```python
from build123d import *

# Parameters (mm, degrees)
SKETCH1_W           = 90
SKETCH1_H           = 145
BOSS_EXTRUDE2_DEPTH = 10
FILLET2_R           = 20
BOSS_EXTRUDE6_DEPTH = 60
CUT_EXTRUDE1_START  = -45
CUT_EXTRUDE1_DEPTH  = 30
SKETCH13_R          = 12
CUT_EXTRUDE2_DEPTH  = 127
BOSS_EXTRUDE8_DEPTH = 10
SKETCH17_R          = 9
CUT_EXTRUDE3_DEPTH  = 20


with BuildPart() as part:
    # Sketch1 → Boss-Extrude2 (new, symmetric)
    with BuildSketch(Plane(origin=(0, 0, 0), x_dir=(1, 0, 0), z_dir=(0, 1, 0))):
        Rectangle(SKETCH1_W, SKETCH1_H)
    extrude(amount=BOSS_EXTRUDE2_DEPTH, both=True)

    # Fillet2
    fillet2_edges = [part.edges().sort_by_distance(p)[0] for p in [
        (45, 0, -72.5),
        (45, 0, 72.5),
        (-45, 0, 72.5),
        (-45, 0, -72.5),
    ]]
    fillet(fillet2_edges, radius=FILLET2_R)

    # Sketch8 → Boss-Extrude6 (add)
    with BuildSketch(Plane(origin=(0, 10, 0), x_dir=(1, 0, 0), z_dir=(0, 1, 0))):
        with BuildLine():
            Line((-34, -7.5), (-34, 42.5))
            ThreePointArc((-34, 42.5), (0, 76.5), (34, 42.5))
            Line((34, 42.5), (34, -7.5))
            Line((34, -7.5), (-34, -7.5))
        make_face()
    extrude(amount=BOSS_EXTRUDE6_DEPTH)

    # Sketch9 → Cut-Extrude1 (cut)
    with BuildSketch(Plane(origin=(0, 70, 0), x_dir=(1, 0, 0), z_dir=(0, 1, 0)).offset(CUT_EXTRUDE1_START)):
        with BuildLine():
            Line((-34, 42.5), (-34, 12.5))
            Line((-34, 12.5), (34, 12.5))
            Line((34, 12.5), (34, 42.5))
            ThreePointArc((34, 42.5), (0, 76.5), (-34, 42.5))
        make_face()
    extrude(amount=CUT_EXTRUDE1_DEPTH, mode=Mode.SUBTRACT)

    # Sketch12 → Revolve1 (revolve)
    with BuildSketch(Plane.XY.offset(-42.5), mode=Mode.PRIVATE) as revolve1_sk:
        Polygon((0, 70), (0, 110), (20, 110), (34, 70), align=None)
    revolve(revolve1_sk.sketch.rotate(Axis((0, 70, -42.5), (0, 1, 0)), 180), axis=Axis((0, 70, -42.5), (0, 1, 0)))

    # Sketch13 → Cut-Extrude2 (cut)
    with BuildSketch(Plane(origin=(0, 110, 0), x_dir=(1, 0, 0), z_dir=(0, 1, 0))):
        with Locations(Location((0, 42.5, 0), (0, 0, 270))):
            Circle(SKETCH13_R)
    extrude(amount=-CUT_EXTRUDE2_DEPTH, mode=Mode.SUBTRACT)

    # Sketch16 → Boss-Extrude8 (add, symmetric)
    with BuildSketch(Plane(origin=(0, 0, 0), x_dir=(0, 0, -1), z_dir=(1, 0, 0))):
        Polygon((-7.5, 70), (-72.5, 10), (-7.5, 10), align=None)
    extrude(amount=BOSS_EXTRUDE8_DEPTH, both=True)

    # Sketch17 → Cut-Extrude3 (cut)
    with BuildSketch(Plane(origin=(0, 10, 0), x_dir=(1, 0, 0), z_dir=(0, 1, 0))):
        with Locations(Location((25, -52.5, 0), (0, 0, 270))):
            Circle(SKETCH17_R)
    cut_extrude3 = extrude(amount=-CUT_EXTRUDE3_DEPTH, mode=Mode.SUBTRACT)

    # Mirror1: Cut-Extrude3 across plane
    add(cut_extrude3.mirror(Plane(origin=(0, 0, 0), x_dir=(0, 0, 1), z_dir=(1, 0, 0))), mode=Mode.SUBTRACT)


solid = part.part
```
For this review, take the finished solid that the model builds, in its own axes (mm). A direction names the side the tool comes from. Round coordinates to 2 decimals unless told otherwise and drop trailing zeros. Write each loop counter-clockwise with the first axis right and the second up, starting at its lowest first coordinate (ties: lowest second). Pieces come first, ordered by that corner, then holes. Notation, with made-up numbers: (26.25, 79) -> (69.25, 79) arc R29 cw to (69.25, 102) -> close; hole circle Ø6 at (10.5, 55.5). An arc over 180 degrees is marked (long way). One line per question, with ' | ' between items. Start each with the question number.
1) Machinability: for faces 4 (the flat face through (-8, 25, -31)), 5 (the flat face through (10, 27, 26)), 6 (the flat face through (-22, 40, 7.5)), which of the approach directions +Z, -Z, +X, -X, +Y, -Y give a long, thin tool a straight path to every point of the face, cutting with its end or side? Answer none if there is none.
2) Add section D-D (x = 37). Write out the cut boundary in (y, z), and give its area (3 significant figures).
3) For pin 1 Ø12 at (x, z) = (-13.5, -61.5) entering from +Y; pin 2 Ø8 at (y, z) = (44.5, 20.5) entering from -X; pin 3 Ø2 at (x, y) = (33.5, 76.5) entering from +Z; pin 4 Ø10 at (x, y) = (-6.5, -0.5) entering from -Z, all flat-tipped, find the tip position at first contact; note any pin that passes through.
4) Add section B-B (y = 17). Write out the cut boundary in (x, z), and give its area (3 significant figures).
5) Mouldability with a two-part tool opening along Z and no side actions: class faces 1 (the flat face through (9, 110, -51)), 2 (the cylindrical face through (0.53, 82.88, -54.49)), 3 (the flat face through (0, 0, -72.5)) as +Z half, -Z half, draft (parallel to the pull), parting line (faces both ways), or undercut.
6) Add section C-C (z = 26). Write out the cut boundary in (x, y), and give its area (3 significant figures).
7) Wall thickness on line 1 along Y through (x, z) = (-15.5, -49.5); line 2 along X through (y, z) = (1.5, 52.5); line 3 along Y through (x, z) = (-15, 15): over which ranges is each line inside the solid? List them lowest first.
8) Add section A-A (x = 0). Write out the cut boundary in (y, z).
Reported:
1) face 4: -Z, +X, -X | face 5: +Z, +X, +Y | face 6: +Z, -X, +Y
2) outline: (-10, -68.5) -> (10, -68.5) -> (10, 68.5) -> (-10, 68.5) -> close | area: 2,740 mm²
3) pin 1: stops at y = 110 | pin 2: stops at x = -10 | pin 3: passes through | pin 4: stops at z = -72.5
4) outline: (-34, -42.5) arc R34 ccw to (34, -42.5) -> (34, 7.5) -> (10, 7.5) -> (10, 64.92) -> (-10, 64.92) -> (-10, 7.5) -> (-34, 7.5) -> close; hole circle Ø24 at (0, -42.5) | area: 5,910 mm²
5) face 1: draft | face 2: undercut | face 3: -Z half
6) outline: (-45, -10) -> (45, -10) -> (45, 10) -> (10, 10) -> (10, 52.92) -> (-10, 52.92) -> (-10, 10) -> (-45, 10) -> close | area: 2,660 mm²
7) line 1: y = -10 to 25, 55 to 110 | line 2: x = -45 to -34, -16 to 16, 34 to 45 | line 3: y = -10 to 10
8) outline: (-10, -72.5) -> (10, -72.5) -> (10, -76.5) -> (25, -76.5) -> (25, -54.5) -> (-10, -54.5) -> close; (-10, -30.5) -> (25, -30.5) -> (25, -12.5) -> (55, -12.5) -> (55, -30.5) -> (110, -30.5) -> (110, -22.5) -> (70, -8.5) -> (70, 7.5) -> (10, 72.5) -> (-10, 72.5) -> close; (55, -76.5) -> (70, -76.5) -> (110, -62.5) -> (110, -54.5) -> (55, -54.5) -> close
